Could you check a few things on this model? Use its own coordinates, in mm. Coordinates: 2 decimals unless noted, no trailing zeros. Loops run counter-clockwise (first coordinate to the right, second up) from the corner with the lowest first, then second, coordinate; pieces in that order, holes last. Notation, with made-up numbers: (8, 2.5) - (62, 2.5) arc R9 cw to (62, 15.5) - close; hole circle Ø9 at (-33.5, 78.5). An arc over 180 degrees is marked (long way). Use CSV: the item, a comma, the result in double quotes.
from build123d import *


with BuildPart() as part:
    # Sketch1 → Revolve1 (revolve)
    with BuildSketch(Plane.XY):
        with BuildLine():
            Line((0, 3.9), (0, 3.7))
            Line((0, 3.7), (0.255, 3.7))
            Line((0.255, 3.7), (0.255, 3.075))
            Line((0.255, 3.075), (0, 3.075))
            Line((0, 3.075), (0, 2.6))
            ThreePointArc((0, 2.6), (0.029289322, 2.529289322), (0.1, 2.5))
            Line((0.1, 2.5), (2.4, 2.5))
            ThreePointArc((2.4, 2.5), (2.470710678, 2.529289322), (2.5, 2.6))
            Line((2.5, 2.6), (2.5, 3.075))
            Line((2.5, 3.075), (2.245, 3.075))
            Line((2.245, 3.075), (2.245, 3.7))
            Line((2.245, 3.7), (2.5, 3.7))
            Line((2.5, 3.7), (2.5, 3.9))
            ThreePointArc((2.5, 3.9), (2.470710678, 3.970710678), (2.4, 4))
            Line((2.4, 4), (0.1, 4))
            ThreePointArc((0.1, 4), (0.029289322, 3.970710678), (0, 3.9))
        make_face()
    revolve(axis=Axis((2.4, 0, 0), (-1, 0, 0)))


solid = part.part
(1) Will these pins go through, and if not, where does the flat tip stop? pin 1 (1 mm diameter, centred on x = 2, z = 2, fed in from +Y); pin 2 (1 mm diameter, centred on x = 2, z = -2.5, fed in from -Y); pin 3 (1 mm diameter, centred on x = 1, y = -1.5, fed in from -Z).
Computed:
pin 1,"stops at y = 3.71"
pin 2,"stops at y = -3.46"
pin 3,"stops at z = -3.87"
(2) Suppose I cut it at C-C (x = 2.1). Write out the boundary of the cut face in (y, z).
Computed:
outline,"circle Ø8 at (0, 0); hole circle Ø5 at (0, 0)"
(3) Thinking about a two-plate mould opening in Z: for faces 1 (the face through (1.27, -0.54, 2.44)), 2 (the face through (1.234, -0.867, 3.905)), which applies, +Z half, -Z half, draft (parallel to the pull), parting line (faces both ways), or undercut?
Computed:
face 1,"undercut"
face 2,"parting line"
(4) Please list where these lines run through material, in increasing order: line 1 (Z direction, x = 2.4, y = 0) (3 decimals); line 2 (Y direction, x = 0.8, z = 0).
Computed:
line 1,"z = -4 to -3.7, -3.075 to -2.5, 2.5 to 3.075, 3.7 to 4"
line 2,"y = -4 to -2.5, 2.5 to 4"
